Autodesk Inventor part; units mm, degrees
ref_plane "YZ Plane" through (0, 0, 0) normal (1, 0, 0) x (0, 1, 0)
ref_plane "XZ Plane" through (0, 0, 0) normal (0, 1, 0) x (-1, 0, 0)
ref_plane "XY Plane" through (0, 0, 0) normal (0, 0, 1) x (1, 0, 0)
sketch "Sketch1" plane through (0, 0, 0) normal (0, 0, 1) x (1, 0, 0)
  line L0 (-15.875, 14.2748) -> (-15.875, -14.2748)
  arc A0 (-14.2748, 15.875) -> (-15.875, 14.2748) centre (-14.2748, 14.2748) ccw
  line L1 (14.2748, 15.875) -> (-14.2748, 15.875)
  arc A1 (15.875, 14.2748) -> (14.2748, 15.875) centre (14.2748, 14.2748) ccw
  line L2 (15.875, -14.2748) -> (15.875, 14.2748)
  arc A2 (14.2748, -15.875) -> (15.875, -14.2748) centre (14.2748, -14.2748) ccw
  line L3 (-14.2748, -15.875) -> (14.2748, -15.875)
  arc A3 (-15.875, -14.2748) -> (-14.2748, -15.875) centre (-14.2748, -14.2748) ccw
  arc A4 (19.05, 15.875) -> (15.875, 19.05) centre (15.875, 15.875) ccw
  line L4 (15.875, 19.05) -> (-15.875, 19.05)
  arc A5 (-15.875, 19.05) -> (-19.05, 15.875) centre (-15.875, 15.875) ccw
  line L5 (-19.05, 15.875) -> (-19.05, -15.875)
  arc A6 (-19.05, -15.875) -> (-15.875, -19.05) centre (-15.875, -15.875) ccw
  line L6 (-15.875, -19.05) -> (15.875, -19.05)
  arc A7 (15.875, -19.05) -> (19.05, -15.875) centre (15.875, -15.875) ccw
  line L7 (19.05, -15.875) -> (19.05, 15.875)
  point P0 (0, 0)
extrude "Extrusion1" add sketch "Sketch1" against normal blind 304.8
properties part number "9700"
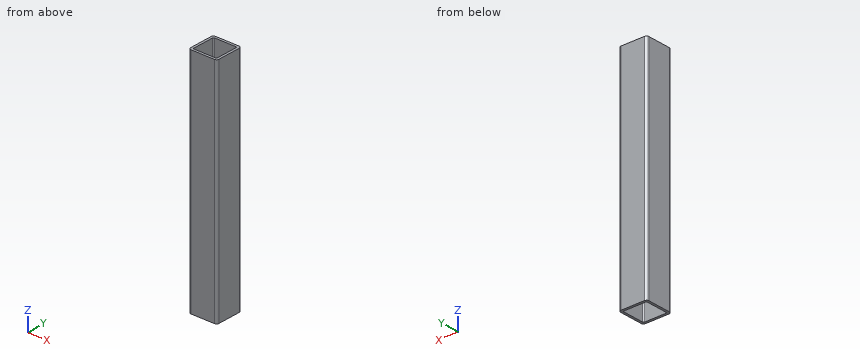
Can you work these out from the model? Positions are in its coordinate system, mm. Round coordinates to 2 decimals unless told otherwise and drop trailing zeros. Order: outer loops, then holes, each group sorted by start corner. A loop starts at its lowest first (then second) coordinate and runs counter-clockwise, first axis right, second up. Notation, with made-up numbers: (48, 20.25) -> (103, 20.25) arc R17 cw to (103, 24.25) -> close; hole circle Ø7 at (46, -11.5). An arc over 180 degrees is marked (long way). Write each question's results on one line, items separated by ' | '. Start each with the question number.
Item 1: If we section it at C-C, the plane z = -122: Write out the boundary of the cut face in (x, y) (3 decimals), then the cut area to 3 significant figures.
Item 2: Please list where these lines run through material, in increasing order: L1, parallel to X at y = 2.5, z = -54 (3 decimals); L2, parallel to Y at x = 15, z = -192.5.
Item 3: If we section it at A-A, the plane x = -4: Write out the boundary of the cut face in (y, z) (3 decimals), then the cut area to 3 significant figures.
Results:
1) outline: (-19.05, -15.875) arc R3.175 ccw to (-15.875, -19.05) -> (15.875, -19.05) arc R3.175 ccw to (19.05, -15.875) -> (19.05, 15.875) arc R3.175 ccw to (15.875, 19.05) -> (-15.875, 19.05) arc R3.175 ccw to (-19.05, 15.875) -> close; hole (-15.875, -14.275) arc R1.6 ccw to (-14.275, -15.875) -> (14.275, -15.875) arc R1.6 ccw to (15.875, -14.275) -> (15.875, 14.275) arc R1.6 ccw to (14.275, 15.875) -> (-14.275, 15.875) arc R1.6 ccw to (-15.875, 14.275) -> close | area: 437 mm2
2) L1: x = -19.05 to -15.875, 15.875 to 19.05 | L2: y = -19.05 to -15.7, 15.7 to 19.05
3) outline: (-19.05, -304.8) -> (-15.875, -304.8) -> (-15.875, 0) -> (-19.05, 0) -> close; (15.875, -304.8) -> (19.05, -304.8) -> (19.05, 0) -> (15.875, 0) -> close | area: 1,940 mm2
